For this review, take the finished solid that the model builds, in its own axes (mm). A direction names the side the tool comes from. Round coordinates to 2 decimals unless told otherwise and drop trailing zeros. Order: outer loops, then holes, each group sorted by start corner. A loop starts at its lowest first (then second) coordinate and runs counter-clockwise, first axis right, second up. Notation, with made-up numbers: (-26, -6) -> (21, -6) arc R22 ccw to (21, 30) -> close; hole circle Ø5 at (19, -27). An arc over 180 degrees is marked (long way). Answer in a Markdown table with one row per item.
```python
from build123d import *

# Parameters (mm, degrees)
SKETCH_1_R          = 15
SKETCH_1_R_2        = 13
EXTRUDE_1_DEPTH     = 10
SKETCH_2_R          = 1
CUT_EXTRUDE_1_DEPTH = 34.301651611


with BuildPart() as part:
    # 草图1 → 凸台-拉伸1 (new body)
    with BuildSketch(Plane(origin=(0, 0, 0), x_dir=(1, 0, 0), z_dir=(0, 1, 0))):
        with Locations(Location((0, 0, 0), (0, 0, 270))):
            Circle(SKETCH_1_R)
        with Locations(Location((0, 0, 0), (0, 0, 270))):
            Circle(SKETCH_1_R_2, mode=Mode.SUBTRACT)
    extrude(amount=EXTRUDE_1_DEPTH)

    # 草图2 → 切除-拉伸1 (cut, through all)
    with BuildSketch(Plane(origin=(0, 0, -13), x_dir=(-1, 0, 0), z_dir=(0, 0, -1))):
        with Locations(Location((0, 5.523046221, 0), (0, 0, 90.000000034))):
            Circle(SKETCH_2_R)
    extrude(amount=-CUT_EXTRUDE_1_DEPTH, mode=Mode.SUBTRACT)


solid = part.part
```
Q1. The part is to be moulded in two halves that separate along Y. For faces 3 (the face through (13.4, 10, -0.1)), 4 (the face through (13.4, 0, -0.1)), 5 (the face through (-0.38, 6.45, 13.97)), say which applies: +Y half, -Y half, draft (parallel to the pull), parting line (faces both ways), or undercut.
Answer key:
| item | result |
|---|---|
| face 3 | +Y half |
| face 4 | -Y half |
| face 5 | undercut |
Q2. Take a section at B-B, the plane x = -8. Write out the cut boundary in (y, z), then the cut area to 3 significant figures.
Answer key:
| item | result |
|---|---|
| outline | (0, -12.69) -> (10, -12.69) -> (10, -10.25) -> (0, -10.25) -> close; (0, 10.25) -> (10, 10.25) -> (10, 12.69) -> (0, 12.69) -> close |
| area | 48.8 mm^2 |
Q3. To check wall thickness, follow probe 1 along X at (y, z) = (4.25, 0); probe 2 along Z at (x, y) = (2.5, 8); probe 3 along X at (y, z) = (7.25, 3.5). State the ranges of each line that lie inside material, in increasing order.
Answer key:
| item | result |
|---|---|
| probe 1 | x = -15 to -13, 13 to 15 |
| probe 2 | z = -14.79 to -12.76, 12.76 to 14.79 |
| probe 3 | x = -14.59 to -12.52, 12.52 to 14.59 |
Q4. Clearance check with flat-ended pins moving along their axes: pin 1 Ø2 at (y, z) = (6.5, -2.5) entering from -X; pin 2 Ø4 at (x, y) = (2.5, 5) entering from +Z; pin 3 Ø0.6 at (x, y) = (0, 5.5) entering from +Z; pin 4 Ø4 at (x, z) = (6, 8) entering from +Y. State where each tip first meets the part, or that it passes through.
Answer key:
| item | result |
|---|---|
| pin 1 | stops at x = -14.92 |
| pin 2 | stops at z = 14.99 |
| pin 3 | stops at z = -13 |
| pin 4 | passes through |
Q5. Tool access review of faces 1 (the face through (0, 6, -13)), 2 (the face through (-5, 5, 12)): name each direction out of +Z, -Z, +X, -X, +Y, -Y from which nothing blocks a thin tool from reaching the whole face with its end or side.
Answer key:
| item | result |
|---|---|
| face 1 | +Z |
| face 2 | +Y, -Y |
Q6. Take a section at A-A, the plane z = 0. Write out the cut boundary in (x, y), then the cut area to 3 significant figures.
Answer key:
| item | result |
|---|---|
| outline | (-15, 0) -> (-13, 0) -> (-13, 10) -> (-15, 10) -> close; (13, 0) -> (15, 0) -> (15, 10) -> (13, 10) -> close |
| area | 40.0 mm^2 |
